Geometry: final body of the model. Coordinates: model frame, mm. A direction names the side the tool comes from. Give positions to 0.01 mm unless a question says otherwise; leave off trailing zeros. Order: outer loops, then holes, each group sorted by start corner. A loop starts at its lowest first (then second) coordinate and runs counter-clockwise, first axis right, second up. Notation, with made-up numbers: M -32.75,-29.75 L 23.25,-29.75 A26 ccw 23.25,-11.75 Z; hole C 22,52.25 d10. An arc over 180 degrees is marked long. Use CSV: the item, a comma, the result in double quotes.
```python
from build123d import *

# Parameters (mm, degrees)
SKETCH1_R                        = 6
BOSS_EXTRUDE1_DEPTH              = 100
BOSS_EXTRUDE1_DEPTH_BACK         = 59
TAP_DRILL_FOR_M5_HELICOIL1_D     = 5.2
TAP_DRILL_FOR_M5_HELICOIL1_DEPTH = 30
TAP_DRILL_FOR_M5_HELICOIL1_TIP   = 1.562237609
TAP_DRILL_FOR_M5_HELICOIL2_D     = 5.2
TAP_DRILL_FOR_M5_HELICOIL2_DEPTH = 30
TAP_DRILL_FOR_M5_HELICOIL2_TIP   = 1.562237609


with BuildPart() as part:
    # Sketch1 → Boss-Extrude1 (new body, two sides)
    with BuildSketch(Plane.XY) as boss_extrude1_sk:
        Circle(SKETCH1_R)
    extrude(amount=BOSS_EXTRUDE1_DEPTH)
    extrude(boss_extrude1_sk.sketch, amount=-BOSS_EXTRUDE1_DEPTH_BACK)

    # Tap Drill for M5 Helicoil1
    with Locations(Plane.XY.offset(100)):
        with Locations((0, 0)):
            Hole(TAP_DRILL_FOR_M5_HELICOIL1_D / 2, depth=TAP_DRILL_FOR_M5_HELICOIL1_DEPTH)
            with Locations((0, 0, -(TAP_DRILL_FOR_M5_HELICOIL1_DEPTH + TAP_DRILL_FOR_M5_HELICOIL1_TIP / 2))):  # 118° drill point
                Cone(0, TAP_DRILL_FOR_M5_HELICOIL1_D / 2, TAP_DRILL_FOR_M5_HELICOIL1_TIP, mode=Mode.SUBTRACT)

    # Tap Drill for M5 Helicoil2
    with Locations(Plane(origin=(0, 0, -59), x_dir=(-1, 0, 0), z_dir=(0, 0, -1))):
        with Locations((0, 0)):
            Hole(TAP_DRILL_FOR_M5_HELICOIL2_D / 2, depth=TAP_DRILL_FOR_M5_HELICOIL2_DEPTH)
            with Locations((0, 0, -(TAP_DRILL_FOR_M5_HELICOIL2_DEPTH + TAP_DRILL_FOR_M5_HELICOIL2_TIP / 2))):  # 118° drill point
                Cone(0, TAP_DRILL_FOR_M5_HELICOIL2_D / 2, TAP_DRILL_FOR_M5_HELICOIL2_TIP, mode=Mode.SUBTRACT)


solid = part.part
```
1. Section C-C, the plane y = -4. Return the cut outline in (x, z).
Answer:
outline,"M -4.47,-59 L 4.47,-59 L 4.47,100 L -4.47,100 Z"
2. Pin query (flat end, axial travel): pin 1 Ø1 at (y, z) = (1.5, 39.5) entering from -X; pin 2 Ø1 at (y, z) = (-2.5, 50) entering from +X; pin 3 Ø3 at (x, y) = (0, 0) entering from +Z. Return the tip coordinate at first contact, or that it passes through.
Answer:
pin 1,"x = -5.92"
pin 2,"x = 5.66"
pin 3,"z = 69.34"
3. Pull-direction query (X, two-part tool) for faces 4 (the face through (-0.36, -0.27, 68.71)), 5 (the face through (-6, 0, 22)), 6 (the face through (3, -1, 100)); classes: +X half, -X half, draft (parallel to the pull), parting line (faces both ways), or undercut.
Answer:
face 4,"undercut"
face 5,"parting line"
face 6,"draft"
4. Reachability of faces 1 (the face through (0.338, 2.578, 84.79)), 2 (the face through (-0.338, 2.578, -43.79)), 3 (the face through (3, -1, -59)) from +Z, -Z, +X, -X, +Y, -Y: full face, straight path, thin tool, end or side. Return the list, or none.
Answer:
face 1,"+Z"
face 2,"-Z"
face 3,"-Z, +X, -X, +Y, -Y"
5. Section B-B, the plane y = 4.5. Return the cut outline in (x, z).
Answer:
outline,"M -3.97,-59 L 3.97,-59 L 3.97,100 L -3.97,100 Z"
6. Line query: line 1 (Y direction, x = 0, z = -41); line 2 (Y direction, x = 1.5, z = 73); line 3 (X direction, y = -0.5, z = -29). Output: solid intervals per line, ascending.
Answer:
line 1,"-6 to -2.6, 2.6 to 6"
line 2,"-5.81 to -2.12, 2.12 to 5.81"
line 3,"-5.98 to -2.55, 2.55 to 5.98"
7. Section A-A, the plane z = 76. Return the cut outline in (x, y).
Answer:
outline,"C 0,0 d12; hole C 0,0 d5.2"
